The model under review builds one solid part; all positions refer to its coordinate system, in mm. A direction names the side the tool comes from. Round coordinates to 2 decimals unless told otherwise and drop trailing zeros. Order: outer loops, then holes, each group sorted by start corner. A loop starts at its lowest first (then second) coordinate and runs counter-clockwise, first axis right, second up.
1) Consider section B-B (z = 75.5). Give the boundary of the cut face in (x, y), then the cut area to 3 significant figures.
2) Clearance check with flat-ended pins moving along their axes: P1, Ø1.5, axis at x = 24, z = 16.5, coming from the +Y side; P2, Ø1.5, axis at x = 10, y = 6, coming from the -Z side. State where each tip first meets the part, or that it passes through.
3) To check wall thickness, follow L1, parallel to Z at x = 20.5, y = 7.5; L2, parallel to Y at x = 18.5, z = 42.5; L3, parallel to Y at x = 7.5, z = 54. State the ranges of each line that lie inside material, in increasing order.
4) Machinability: for faces 4 (the face through (10.77, 5.49, 79.01)), 5 (the face through (18, 8, 2)), 6 (the face through (1.374, 2.074, 40.56)), 7 (the face through (17.199, 9.453, 0.986)), which of the approach directions +Z, -Z, +X, -X, +Y, -Y give a long, thin tool a straight path to every point of the face, cutting with its end or side? Answer none if there is none.
5) Consider section C-C (x = 17.5). Give the boundary of the cut face in (y, z), then the cut area to 3 significant figures.
6) Consider section D-D (y = 5.5). Give the boundary of the cut face in (x, z), then the cut area to 3 significant figures.
7) Consider section A-A (y = 1.5). Give the boundary of the cut face in (x, z).
8) Mouldability with a two-part tool opening along X and no side actions: class faces 1 (the face through (18, 8, 78)), 2 (the face through (10.77, 5.49, 1.01)), 3 (the face through (24.866, 10.624, 1.014)) as pulls with the +X half, pulls with the -X half, needs draft (parallel to the pull), parting line crosses it, or undercut.
from build123d import *

# Parameters (mm, degrees)
BOSS_EXTRUDE1_DEPTH = 80
SKETCH2_W           = 2
SKETCH2_H           = 80
SKETCH2_W_2         = 15
SKETCH2_H_2         = 2
BOSS_EXTRUDE2_DEPTH = 3


with BuildPart() as part:
    # Sketch1 → Boss-Extrude1 (new body)
    with BuildSketch(Plane.XY):
        Polygon((0, 0), (30, 0), (30, 10.919107028), align=None)
    extrude(amount=BOSS_EXTRUDE1_DEPTH)

    # Sketch2 → Boss-Extrude2 (add)
    with BuildSketch(Plane(origin=(0, 0, 0), x_dir=(0.9396926207859082, 0.34202014332566943, 0), z_dir=(-0.34202014332566943, 0.9396926207859082, 0))):
        with Locations((1, -40)):
            Rectangle(SKETCH2_W, SKETCH2_H)
        with Locations((19.5, -1)):
            Rectangle(SKETCH2_W_2, SKETCH2_H_2)
        with Locations((19.5, -79)):
            Rectangle(SKETCH2_W_2, SKETCH2_H_2)
    extrude(amount=BOSS_EXTRUDE2_DEPTH)


solid = part.part
Answer below:
1. outline: (-1.03, 2.82) - (0, 0) - (30, 0) - (30, 10.92) - (1.88, 0.68) - (0.85, 3.5) - close
1. area: 170 mm2
2. P1: stops at y = 9.01
2. P2: stops at z = 0
3. L1: z = 0 to 2, 78 to 80
3. L2: y = 0 to 6.73
3. L3: y = 0 to 2.73
4. face 4: +Z, -Z, -X
4. face 5: -X, +Y
4. face 6: +Z, -Z, +Y
4. face 7: +Z, -Z, -X, +Y
5. outline: (0, 0) - (9.56, 0) - (9.56, 2) - (6.37, 2) - (6.37, 78) - (9.56, 78) - (9.56, 80) - (0, 80) - close
5. area: 522 mm2
6. outline: (10.77, 0) - (30, 0) - (30, 80) - (10.77, 80) - (10.77, 78) - (15.11, 78) - (15.11, 2) - (10.77, 2) - close
6. area: 1,210 mm2
7. outline: (-0.55, 0) - (1.58, 0) - (1.58, 80) - (-0.55, 80) - close; (4.12, 0) - (30, 0) - (30, 80) - (4.12, 80) - close
8. face 1: needs draft
8. face 2: pulls with the -X half
8. face 3: undercut
